Verification items for this drawing (mm, ordinates from the low corner). A direction names the side the tool comes from. Round coordinates to 2 decimals unless told otherwise and drop trailing zeros. Loops run counter-clockwise (first coordinate to the right, second up) from the corner with the lowest first, then second, coordinate; pieces in that order, holes last. Notation, with made-up numbers: M -2,61 L 45,61 A23 ccw 45,71 Z; hole C 55,14.5 d10. An arc over 180 degrees is marked long. Write item = value, one per line. Start each with the question number.
(1) Scan lines: L1, parallel to X at y = 19.5, z = 3.5 (1 decimal); L2, parallel to Z at x = 8.5, y = 73.5 (1 decimal). Record each from-to range of solid material in increasing order. Write a range as from..to.
(2) Go/stop test with a flat-tipped pin: P1, Ø10, axis at x = 42, y = 55.5, coming from the +Z side (1 decimal). Record where the tip stops, or that it passes through.
(3) Set-up check for the marked faces 1 and 2: record each of +Z, -Z, +X, -X, +Y, -Y from which the full face is reachable in a straight line by a thin tool's end or side.
(4) Cross-section at A-A on z = 5. Record the boundary of the cut face in (x, y) (1 decimal), plus the area to 3 significant figures.
(5) Cross-section at B-B on y = 75. Record the boundary of the cut face in (x, z) (1 decimal).
(6) Mould release check, pull along X, two halves, no side actions. Record for the marked faces 3, 4 and 5: pulls with the +X half, pulls with the -X half, needs draft (parallel to the pull), parting line crosses it, or undercut.
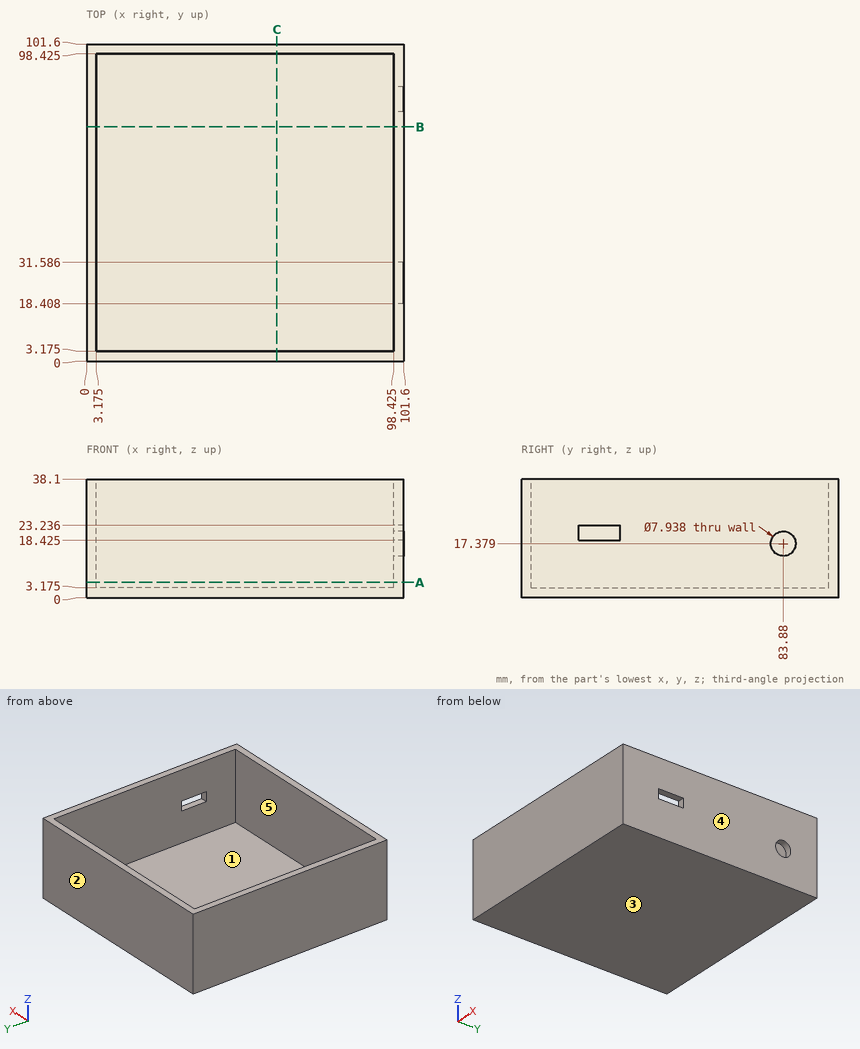
Result:
q1.L1 = 0..3.2, 98.4..101.6
q1.L2 = 0..3.2
q2.P1 = 3.2
q3.face_1 = +Z
q3.face_2 = +Z, -Z, +X, -X, +Y
q4.outline = M 0,0 L 101.6,0 L 101.6,101.6 L 0,101.6 Z; hole M 3.2,3.2 L 98.4,3.2 L 98.4,98.4 L 3.2,98.4 Z
q4.area = 1,250 mm^2
q5.outline = M 0,0 L 101.6,0 L 101.6,38.1 L 98.4,38.1 L 98.4,3.2 L 3.2,3.2 L 3.2,38.1 L 0,38.1 Z
q6.face_3 = needs draft
q6.face_4 = pulls with the +X half
q6.face_5 = undercut
